```python
from build123d import *

# Parameters (mm, degrees)
BOSS_EXTRUDE1_DEPTH = 15
SKETCH2_R           = 3.5
CUT_EXTRUDE1_DEPTH  = 46
SKETCH3_R           = 3.5
CUT_EXTRUDE2_DEPTH  = 46


with BuildPart() as part:
    # Sketch1 → Boss-Extrude1 (new, symmetric)
    with BuildSketch(Plane.XY):
        with BuildLine():
            Line((0, 0), (0, 30))
            ThreePointArc((0, 30), (3.535533906, 28.535533906), (5, 25))
            Line((5, 25), (5, 10))
            ThreePointArc((5, 10), (6.464466094, 6.464466094), (10, 5))
            Line((10, 5), (25, 5))
            ThreePointArc((25, 5), (28.535533906, 3.535533906), (30, 0))
            Line((30, 0), (0, 0))
        make_face()
    extrude(amount=BOSS_EXTRUDE1_DEPTH, both=True)

    # Sketch2 → Cut-Extrude1 (cut, through all)
    with BuildSketch(Plane(origin=(0, 0, 0), x_dir=(1, 0, 0), z_dir=(0, 1, 0))):
        with Locations((15, 0)):
            Circle(SKETCH2_R)
    extrude(amount=CUT_EXTRUDE1_DEPTH, mode=Mode.SUBTRACT)

    # Sketch3 → Cut-Extrude2 (cut, through all)
    with BuildSketch(Plane(origin=(0, 0, 0), x_dir=(0, 0, -1), z_dir=(1, 0, 0))):
        with Locations(Location((0, 15, 0), (0, 0, 270))):
            Circle(SKETCH3_R)
    extrude(amount=CUT_EXTRUDE2_DEPTH, mode=Mode.SUBTRACT)


solid = part.part
```
CAD build for the part. Positions are in the model's coordinates, mm. A direction names the side the tool comes from. Round coordinates to 2 decimals unless told otherwise and drop trailing zeros. Write each loop counter-clockwise with the first axis right and the second up, starting at its lowest first coordinate (ties: lowest second). Pieces come first, ordered by that corner, then holes.
Item 1: Band-saw the part on A-A on z = 0. Write the cut outline in (x, y), then the cut area to 3 significant figures.
Filled in:
outline: (0, 0) - (11.5, 0) - (11.5, 5) - (10, 5) arc R5 cw to (5, 10) - (5, 11.5) - (0, 11.5) - close; (0, 18.5) - (5, 18.5) - (5, 25) arc R5 ccw to (0, 30) - close; (18.5, 0) - (30, 0) arc R5 ccw to (25, 5) - (18.5, 5) - close
area: 200 mm2
Item 2: Drop flat-ended pins along their axis: pin 1 Ø12 at (x, y) = (14, 18) entering from -Z; pin 2 Ø3 at (y, z) = (23, 2.5) entering from +X; pin 3 Ø1 at (y, z) = (26.5, -10.5) entering from +X; pin 4 Ø10 at (y, z) = (12.5, 0) entering from +X. Give the stop position or say it passes through.
Filled in:
pin 1: passes through
pin 2: stops at x = 5
pin 3: stops at x = 4.9
pin 4: stops at x = 5.67
Item 3: Mould opens along Y. For faces 3 (the flat face through (19, 0, 0)), 4 (the cylindrical face through (2.465, 11.767, 1.341)), 5 (the flat face through (19, 5, 0)), 6 (the flat face through (6, 6, 15)) say: released by +Y, released by -Y, zero draft, split by the parting line, or undercut.
Filled in:
face 3: released by -Y
face 4: undercut
face 5: released by +Y
face 6: zero draft
Item 4: Band-saw the part on B-B on x = 15. Write the cut outline in (y, z), then the cut area to 3 significant figures.
Filled in:
outline: (0, -15) - (5, -15) - (5, -3.5) - (0, -3.5) - close; (0, 3.5) - (5, 3.5) - (5, 15) - (0, 15) - close
area: 115 mm2
Item 5: Tool access for faces 1 (the flat face through (0, 11, 0)), 2 (the flat face through (5, 19, 0)): list every direction of +Z, -Z, +X, -X, +Y, -Y with a clear straight run to the whole face (end or side of a thin tool).
Filled in:
face 1: +Z, -Z, -X, +Y, -Y
face 2: +Z, -Z, +X, +Y
Item 6: Band-saw the part on D-D on z = 8. Write the cut outline in (x, y).
Filled in:
outline: (0, 0) - (30, 0) arc R5 ccw to (25, 5) - (10, 5) arc R5 cw to (5, 10) - (5, 25) arc R5 ccw to (0, 30) - close
Item 7: Drill centre lines: L1, parallel to Z at x = 15, y = 2; L2, parallel to Y at x = 23, z = -3.75. Where is each one in solid material? Low to high.
Filled in:
L1: z = -15 to -3.5, 3.5 to 15
L2: y = 0 to 5
